Here's the drawing with two shaded views (mm, measured from the low corner). I have some questions. Coordinates: 2 decimals unless noted, no trailing zeros. Loops run counter-clockwise (first coordinate to the right, second up) from the corner with the lowest first, then second, coordinate; pieces in that order, holes last.
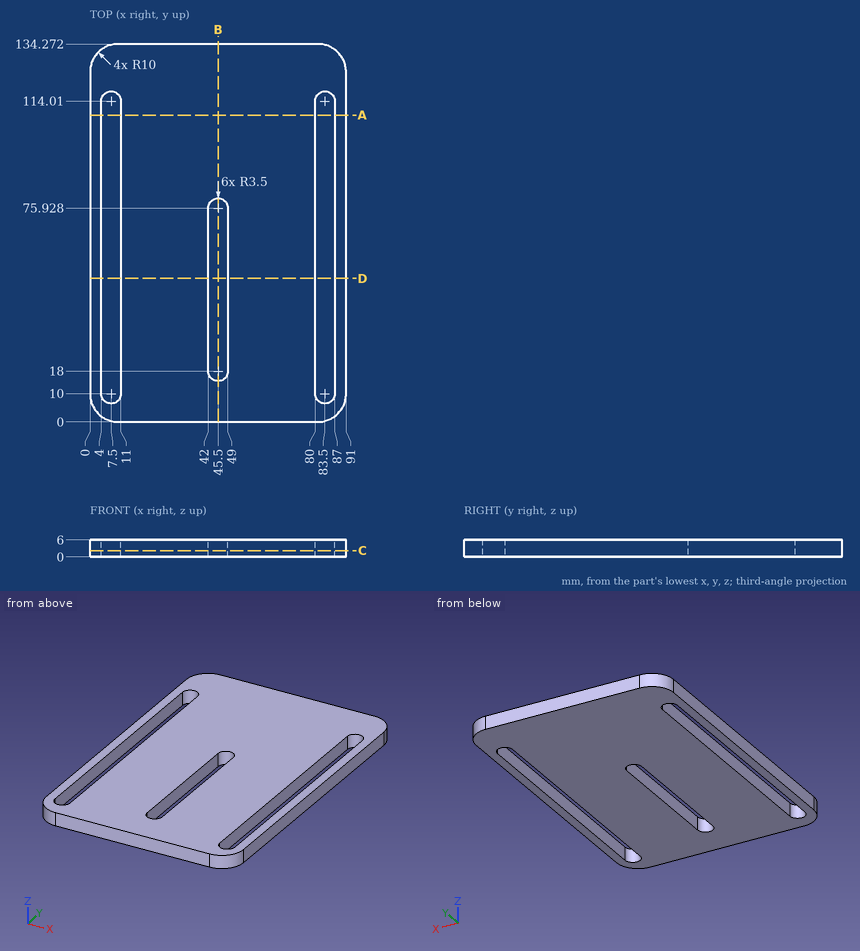
(1) I want a section at B-B on x = 45.5. Write out the boundary of the cut face in (y, z), then the cut area to 3 significant figures.
Check values:
outline: (0, 0) - (14.5, 0) - (14.5, 6) - (0, 6) - close; (79.43, 0) - (134.27, 0) - (134.27, 6) - (79.43, 6) - close
area: 416 mm2
(2) I want a section at D-D on y = 51. Write out the boundary of the cut face in (x, z), then the cut area to 3 significant figures.
Check values:
outline: (0, 0) - (4, 0) - (4, 6) - (0, 6) - close; (11, 0) - (42, 0) - (42, 6) - (11, 6) - close; (49, 0) - (80, 0) - (80, 6) - (49, 6) - close; (87, 0) - (91, 0) - (91, 6) - (87, 6) - close
area: 420 mm2
(3) I'm going to push a flat-ended pin straight in: pin 1 (3 mm diameter, centred on x = 68.5, y = 82, fed in from -Z). Where does the tip first touch, or does it pass through?
Check values:
pin 1: stops at z = 0
(4) I want a section at C-C on z = 2.15. Write out the boundary of the cut face in (x, y).
Check values:
outline: (0, 10) arc R10 ccw to (10, 0) - (81, 0) arc R10 ccw to (91, 10) - (91, 124.27) arc R10 ccw to (81, 134.27) - (10, 134.27) arc R10 ccw to (0, 124.27) - close; hole (4, 10) arc R3.5 ccw to (11, 10) - (11, 114.01) arc R3.5 ccw to (4, 114.01) - close; hole (42, 18) arc R3.5 ccw to (49, 18) - (49, 75.93) arc R3.5 ccw to (42, 75.93) - close; hole (80, 10) arc R3.5 ccw to (87, 10) - (87, 114.01) arc R3.5 ccw to (80, 114.01) - close
(5) If I drill on probe 1 along X at (y, z) = (31.5, 1.65); probe 2 along X at (y, z) = (105.5, 5.35); probe 3 along Y at (x, z) = (84, 3.9) (1 decimal), over which ranges is the centre line in solid material (lowest first)?
Check values:
probe 1: x = 0 to 4, 11 to 42, 49 to 80, 87 to 91
probe 2: x = 0 to 4, 11 to 80, 87 to 91
probe 3: y = 0.5 to 6.5, 117.5 to 133.8
(6) I want a section at A-A on y = 109. Write out the boundary of the cut face in (x, z).
Check values:
outline: (0, 0) - (4, 0) - (4, 6) - (0, 6) - close; (11, 0) - (80, 0) - (80, 6) - (11, 6) - close; (87, 0) - (91, 0) - (91, 6) - (87, 6) - close
